Input: dimensioned drawing with shaded views. Units: mm. Origin: part minimum x, y, z. A direction names the side the tool comes from. Round coordinates to 2 decimals unless told otherwise and drop trailing zeros. Order: outer loops, then holes, each group sorted by start corner. A loop starts at its lowest first (then second) coordinate and runs counter-clockwise, first axis right, second up. Notation, with made-up numbers: M -1.5,40 L 14.5,40 A23 cw 14.5,76 Z; hole C 75,-6.5 d7. An arc over 180 degrees is marked long. Answer as CSV lines item,"result". Start each with the question number.
Item 1: Pull-direction query (X, two-part tool) for the marked faces 1, 2 and 3; classes: +X half, -X half, draft (parallel to the pull), parting line (faces both ways), or undercut.
Item 2: Section query C-C on y = 3.5. State how many separate pieces and enclosed holes the cut face has, plus the area to 3 significant figures.
Item 3: Set-up query: the marked faces 4 and 5. Return all of +Z, -Z, +X, -X, +Y, -Y with unobstructed straight access to the full face (end or side cutting, diameter ignored); none if empty.
Item 4: Line query: line 1 (Z direction, x = 30, y = 2.5); line 2 (Z direction, x = 30, y = 1). Output: solid intervals per line, ascending. Write a range as [from, to].
Item 5: Section query D-D on z = 23.5. Return the cut outline in (x, y), plus the area to 3 significant figures.
Item 6: Section query B-B on z = 30. Return the cut outline in (x, y), plus the area to 3 significant figures.
Item 7: First-contact query: P1, Ø11, axis at x = 26, z = 34, coming from the -Y side; P2, Ø3, axis at x = 51.92, z = 30, coming from the +Y side; P3, Ø4.5, axis at x = 30, z = 8.08, coming from the +Y side. Flat tips, straight axial feed; report the tip coordinate or a pass-through.
Item 8: Section query A-A on x = 30. Return the cut outline in (y, z).
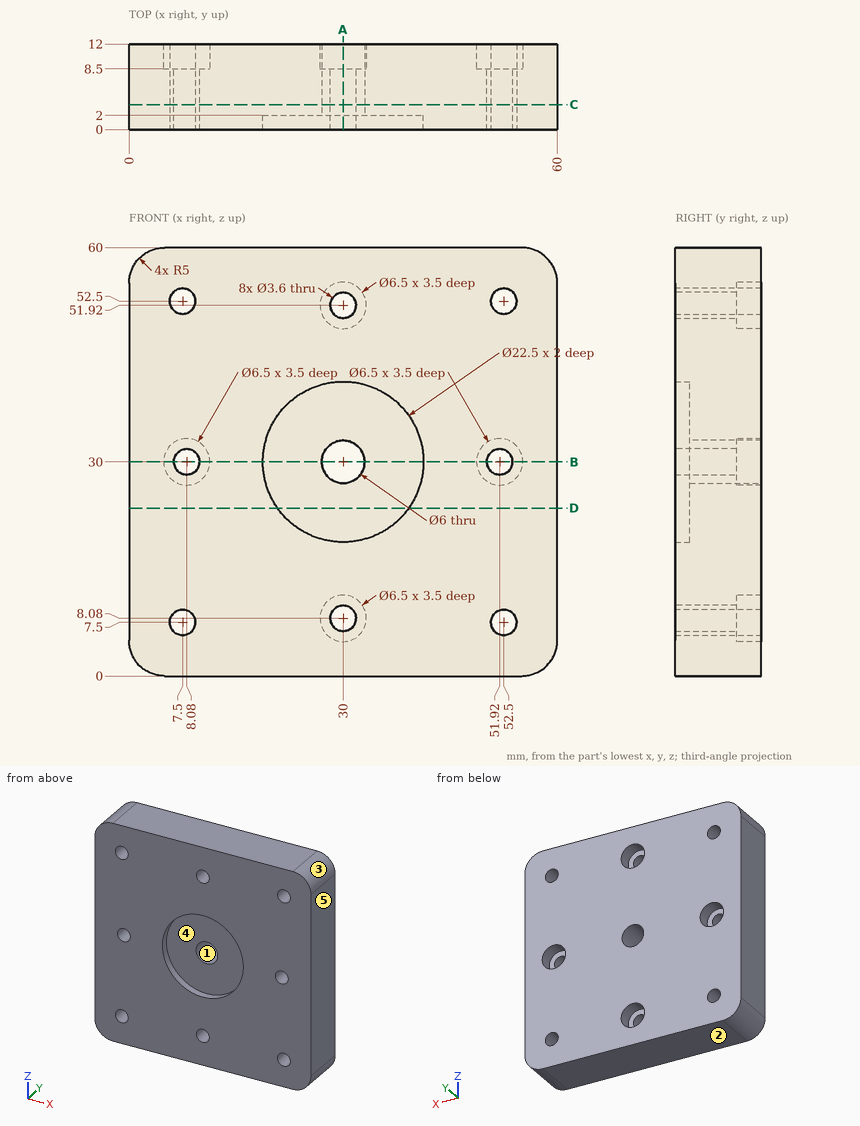
Results:
1,face 1,"undercut"
1,face 2,"draft"
1,face 3,"+X half"
2,separate pieces,"1"
2,enclosed holes,"9"
2,area,"3,470 mm^2"
3,face 4,"-Y"
3,face 5,"+Z, -Z, +X, +Y, -Y"
4,line 1,"[0, 6.28], [9.88, 27], [33, 50.12], [53.72, 60]"
4,line 2,"[0, 6.28], [9.88, 18.75], [41.25, 50.12], [53.72, 60]"
5,outline,"M 0,0 L 20.82,0 L 20.82,2 L 39.18,2 L 39.18,0 L 60,0 L 60,12 L 0,12 Z"
5,area,"683 mm^2"
6,outline,"M 0,0 L 6.28,0 L 6.28,8.5 L 4.83,8.5 L 4.83,12 L 0,12 Z; M 9.88,0 L 18.75,0 L 18.75,2 L 27,2 L 27,12 L 11.33,12 L 11.33,8.5 L 9.88,8.5 Z; M 33,2 L 41.25,2 L 41.25,0 L 50.12,0 L 50.12,8.5 L 48.67,8.5 L 48.67,12 L 33,12 Z; M 53.72,0 L 60,0 L 60,12 L 55.17,12 L 55.17,8.5 L 53.72,8.5 Z"
6,area,"508 mm^2"
7,P1,"y = 2"
7,P2,"through"
7,P3,"y = 8.5"
8,outline,"M 0,0 L 12,0 L 12,4.83 L 8.5,4.83 L 8.5,6.28 L 0,6.28 Z; M 0,9.88 L 8.5,9.88 L 8.5,11.33 L 12,11.33 L 12,27 L 2,27 L 2,18.75 L 0,18.75 Z; M 0,41.25 L 2,41.25 L 2,33 L 12,33 L 12,48.67 L 8.5,48.67 L 8.5,50.12 L 0,50.12 Z; M 0,53.72 L 8.5,53.72 L 8.5,55.17 L 12,55.17 L 12,60 L 0,60 Z"
